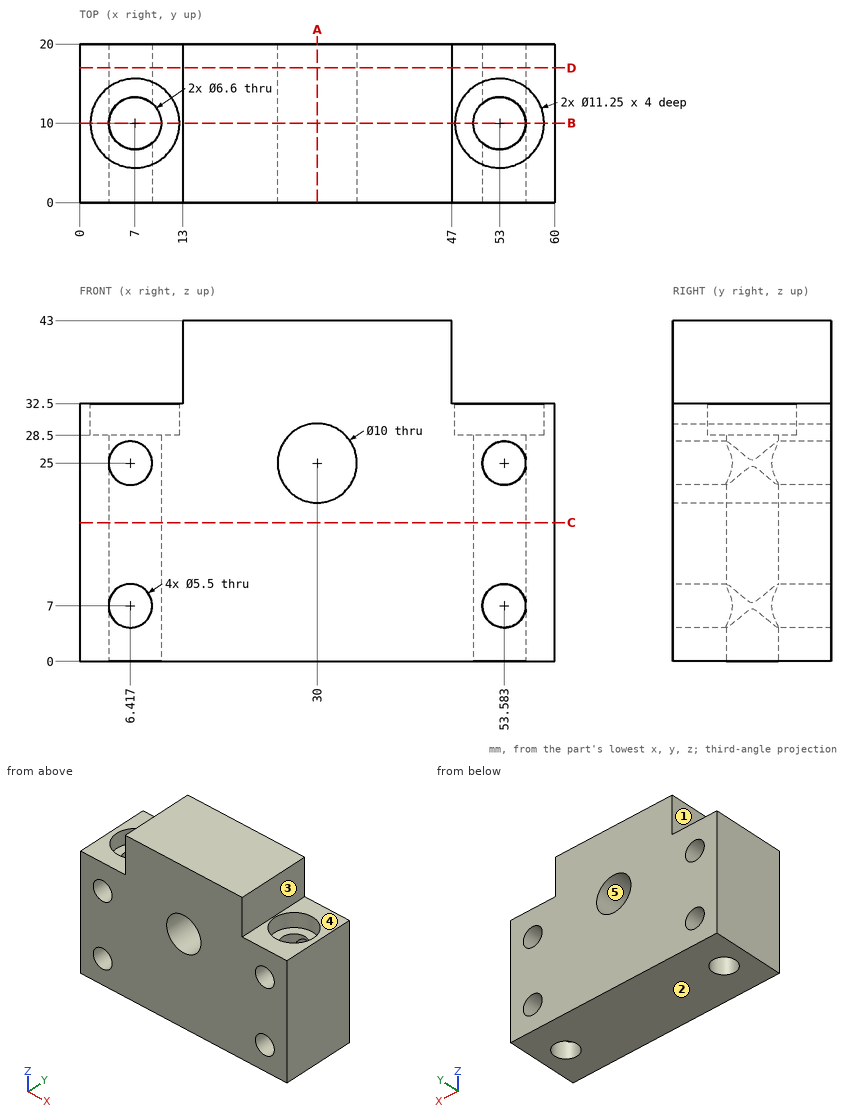
Study the drawing (mm; zero at the part's minimum x, y, z) and answer. A direction names the side the tool comes from. Give positions to 0.01 mm unless a question says otherwise; leave off trailing zeros. Write each loop counter-clockwise with the first axis right and the second up, starting at its lowest first coordinate (ties: lowest second). Pieces come first, ordered by that corner, then holes. Notation, with made-up numbers: (9, 33.25) - (20, 33.25) arc R20 cw to (20, 59.25) - close; hole circle Ø1 at (-0.5, 44). An arc over 180 degrees is marked (long way). One line per question, with ' | ' between items. Start each with the question number.
1. Determine the mould class of the marked faces 3, 4 and 5 for opening direction X: +X half, -X half, draft (parallel to the pull), parting line (faces both ways), or undercut.
2. Section D-D, the plane y = 17 is taken. Determine the outline of the cut face in (x, z).
3. Given P1, Ø5, axis at y = 12.5, z = 38, coming from the -X side; P2, Ø9, axis at x = 54.5, y = 8, coming from the +Z side; P3, Ø3, axis at y = 8, z = 35.5, coming from the +X side, each flat-ended and moving along its own axis, determine where each tip first touches the part or whether it passes through.
4. Section B-B, the plane y = 10 is taken. Count the separate pieces of the cut face and the enclosed holes in it, then the cut area to 3 significant figures.
5. Straight lines are drawn through the part: line 1 (Z direction, x = 53.5, y = 4.75); line 2 (Y direction, x = 7, z = 30.1) (1 decimal); line 3 (X direction, y = 11, z = 15) (1 decimal). For each, find the intervals that lie inside material, in ascending order.
6. Section C-C, the plane z = 17.5 is taken. Determine the outline of the cut face in (x, y), then the cut area to 3 significant figures.
7. For the marked faces 1 and 2, determine the directions among +Z, -Z, +X, -X, +Y, -Y from which every point of the face is accessible in a straight line to the end or side of a thin tool.
8. Section A-A, the plane x = 30 is taken. Determine the outline of the cut face in (y, z).
Result:
1) face 3: +X half | face 4: draft | face 5: undercut
2) outline: (0, 0) - (60, 0) - (60, 32.5) - (47, 32.5) - (47, 43) - (13, 43) - (13, 32.5) - (0, 32.5) - close; hole circle Ø5.5 at (6.42, 7); hole circle Ø5.5 at (6.42, 25); hole circle Ø10 at (30, 25); hole circle Ø5.5 at (53.58, 7); hole circle Ø5.5 at (53.58, 25)
3) P1: stops at x = 13 | P2: stops at z = 32.5 | P3: stops at x = 47
4) separate pieces: 3 | enclosed holes: 1 | area: 1,760 mm2
5) line 1: z = 0 to 4.25, 9.75 to 22.25, 27.75 to 28.5 | line 2: y = 0 to 4.4, 15.6 to 20 | line 3: x = 0 to 3.9, 10.1 to 49.9, 56.1 to 60
6) outline: (0, 0) - (60, 0) - (60, 20) - (0, 20) - close; hole circle Ø6.6 at (7, 10); hole circle Ø6.6 at (53, 10) | area: 1,130 mm2
7) face 1: +Z, -X, +Y, -Y | face 2: -Z, +X, -X, +Y, -Y
8) outline: (0, 0) - (20, 0) - (20, 20) - (0, 20) - close; (0, 30) - (20, 30) - (20, 43) - (0, 43) - close
